```python
from build123d import *
from build123d.topology import SkipClean

# Parameters (mm, degrees)
SALIENTE_EXTRUIR1_REACH      = 49.713
SALIENTE_EXTRUIR1_END_RADIUS = 16
SALIENTE_EXTRUIR1_START      = -20
CROQUIS2_R                   = 7.5


with BuildPart() as part:
    # Croquis1 → Revolución-Lámina1 (revolve)
    with BuildSketch(Plane.XY):
        with BuildLine():
            ThreePointArc((15, 0), (10.606601718, 10.606601718), (0, 15))
            Line((0, 15), (0, 16))
            ThreePointArc((0, 16), (11.313708499, 11.313708499), (16, 0))
            Line((16, 0), (15, 0))
        make_face()
    revolve(axis=Axis((0, 0, 0), (1, 0, 0)))

    # Saliente-Extruir1: up to this sphere (the profile starts outside it)
    with SkipClean():  # the faces are left unmerged after this step: merging them gives an invalid solid
        saliente_extruir1_end = Location((0, 0, 0)) * Sphere(SALIENTE_EXTRUIR1_END_RADIUS, mode=Mode.PRIVATE)
        # Croquis2 → Saliente-Extruir1 (add, up to the surface)
        with BuildSketch(Plane.ZY.offset(SALIENTE_EXTRUIR1_START), mode=Mode.PRIVATE) as saliente_extruir1_sk1:
            Circle(CROQUIS2_R)
        saliente_extruir1_tool1 = extrude(saliente_extruir1_sk1.sketch, amount=SALIENTE_EXTRUIR1_REACH, mode=Mode.PRIVATE) - saliente_extruir1_end
        add(saliente_extruir1_tool1.solids().sort_by_distance((20, 0, 0))[0])

    # Croquis5 → Revolución1 (revolve)
    with BuildSketch(Plane.XY, mode=Mode.PRIVATE) as revoluci_n1_sk:
        with BuildLine():
            Line((20, 7.5), (20, 0))
            Line((20, 0), (47.990381057, 0))
            ThreePointArc((47.990381057, 0), (43.596982775, 10.606601718), (32.990381057, 15))
            ThreePointArc((32.990381057, 15), (25.490381057, 12.990381057), (20, 7.5))
        make_face()
    revolve(revoluci_n1_sk.sketch.rotate(Axis((20, 0, 0), (1, 0, 0)), 90), axis=Axis((20, 0, 0), (1, 0, 0)))


solid = part.part
```
CAD build for the part. Positions are in the model's coordinates, mm. Round coordinates to 2 decimals unless told otherwise and drop trailing zeros. Loops run counter-clockwise (first coordinate to the right, second up) from the corner with the lowest first, then second, coordinate; pieces in that order, holes last. Notation, with made-up numbers: (71.25, -40) - (106.25, -40) arc R21 ccw to (106.25, -13) - close; hole circle Ø10 at (-32.5, -34). An arc over 180 degrees is marked (long way). Return JSON: item names as keys, results as strings. Group by question number.
Q1. Flat gauge pins, fed straight in: pin 1 Ø3 at (x, y) = (22.5, 1.5) entering from +Z; pin 2 Ø12 at (y, z) = (-6.5, 3.5) entering from +X; pin 3 Ø5 at (y, z) = (8, 7) entering from -X. Where does each tip first touch, or does it go through?
Q2. Band-saw the part on B-B on z = -10. Give the cut face in (x, y).
Q3. Band-saw the part on A-A on y = 0. Give the cut face in (x, z), plus the area to 3 significant figures.
Q4. Band-saw the part on C-C on y = -9.5. Give the cut face in (x, z).
Q5. Drill centre lines: line 1 along Y through (x, z) = (6.5, -7); line 2 along X through (y, z) = (-1.5, -13.5); line 3 along Z through (x, y) = (9, -2.5). Where is each one in solid material? Low to high. Write a range as [from, to].
Solutions:
{
 "1": {"pin 1": "stops at z = 11.93", "pin 2": "stops at x = 47.93", "pin 3": "stops at x = 7.25"},
 "2": {"outline": "(0, -12.49) arc R12.49 ccw to (0, 12.49) - (0, 11.18) arc R11.18 cw to (0, -11.18) - close; circle Ø22.36 at (32.99, 0)"},
 "3": {"outline": "(0, -16) arc R16 ccw to (14.13, -7.5) - (20, -7.5) arc R15 ccw (long way) to (20, 7.5) - (14.13, 7.5) arc R16 ccw to (0, 16) - (0, 15) arc R15 cw to (0, -15) - close", "area": "804 mm^2"},
 "4": {"outline": "(0, -12.87) arc R12.87 ccw to (0, 12.87) - (0, 11.61) arc R11.61 cw to (0, -11.61) - close; circle Ø23.22 at (32.99, 0)"},
 "5": {"line 1": "y = [-12.84, -11.57], [11.57, 12.84]", "line 2": "x = [6.36, 8.46], [26.63, 39.35]", "line 3": "z = [-12.99, -11.74], [11.74, 12.99]"}
}
